The listing builds one solid part. Answer for the finished solid, in the listing's coordinates (mm). Face numbers are marked on the shaded views. A direction names the side the tool comes from. Give positions to 0.01 mm unless a question says otherwise; leave off trailing zeros. Write each loop counter-clockwise with the first axis right and the second up, starting at its lowest first coordinate (ties: lowest second). Pieces come first, ordered by that corner, then holes. Notation, with made-up numbers: (6.5, -20) -> (41.5, -20) arc R13 ccw to (41.5, -11) -> close; hole circle Ø11 at (21, -38.5). An arc over 180 degrees is marked (long way). Use CSV: the item, a comma, the result in double quotes. Start each with the question number.
from build123d import *

# Parameters (mm, degrees)
BASE_EXTRUDE_DEPTH      = 38.1
SKETCH2_R               = 2.3495
MOTOR_HOLE_CUT_DEPTH    = 48.603828628
SKETCH3_R               = 2.3495
MOUNTING_HOLE_CUT_DEPTH = 47.6627796
CORNER_FILLETS_R        = 6.35


with BuildPart() as part:
    # Sketch1 → Base Extrude (new body)
    with BuildSketch(Plane(origin=(0, 0, 0), x_dir=(1, 0, 0), z_dir=(0, 1, 0))):
        Polygon((0, 0), (24.13, 0), (24.13, -3.81), (11.7475, -3.81), (5.08, -6.6548), (5.08, -19.05), (0, -19.05), align=None)
    extrude(amount=BASE_EXTRUDE_DEPTH)

    # Sketch2 → Motor Hole Cut (cut, through all)
    with BuildSketch(Plane.XY.offset(3.81)):
        with Locations((17.697323232, 6.35)):
            Circle(SKETCH2_R)
        with Locations((17.78, 19.05)):
            Circle(SKETCH2_R)
        with Locations((17.78, 31.75)):
            Circle(SKETCH2_R)
    extrude(amount=-MOTOR_HOLE_CUT_DEPTH, mode=Mode.SUBTRACT)

    # Sketch3 → Mounting Hole Cut (cut, through all)
    with BuildSketch(Plane(origin=(5.08, 0, 0), x_dir=(0, 0, -1), z_dir=(1, 0, 0))):
        with Locations((-12.7, 31.75)):
            Circle(SKETCH3_R)
        with Locations((-12.7, 19.05)):
            Circle(SKETCH3_R)
        with Locations((-12.7, 6.35)):
            Circle(SKETCH3_R)
    extrude(amount=-MOUNTING_HOLE_CUT_DEPTH, mode=Mode.SUBTRACT)

    # Corner Fillets
    corner_fillets_edges = [part.edges().sort_by_distance(p)[0] for p in [
        (24.13, 38.1, 1.905),
        (24.13, 0, 1.905),
        (2.54, 38.1, 19.05),
        (2.54, 0, 19.05),
    ]]
    fillet(corner_fillets_edges, radius=CORNER_FILLETS_R)


solid = part.part
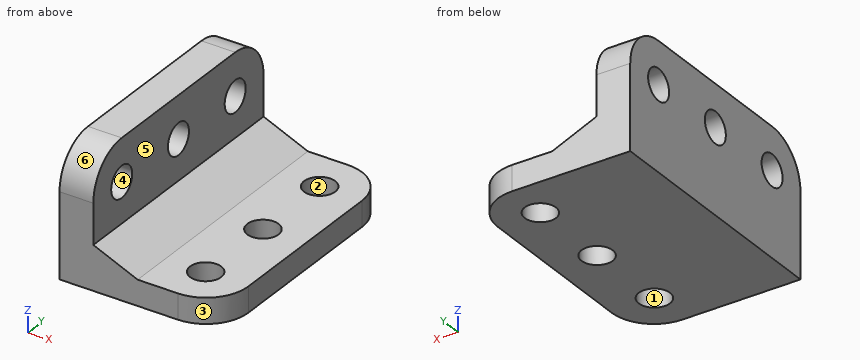
Q1. Section A-A on y = 19.05 is taken. Give the vertices of the cut face in (x, z), then the cut area to 3 significant figures.
Q2. For the marked faces 5 and 6, determine the directions among +Z, -Z, +X, -X, +Y, -Y from which every point of the face is accessible in a straight line to the end or side of a thin tool.
Q3. The mould has two halves that part along X. Classify the marked faces 1, 2, 3 and 4: +X half, -X half, draft (parallel to the pull), parting line (faces both ways), or undercut.
Q4. Section B-B on x = 3 is taken. Give the vertices of the cut face in (y, z), then the cut area to 3 significant figures.
Q5. Flat-ended cylindrical pins translate along their axes: pin 1 Ø3 at (y, z) = (26, 16) entering from +X; pin 2 Ø8 at (y, z) = (30, 8.5) entering from +X; pin 3 Ø5.5 at (x, y) = (17.78, 31.75) entering from +Z; pin 4 Ø4 at (y, z) = (6.35, 12.7) entering from -X. Find the tip coordinate at first contact, or state that the pin passes through.
Q6. Section D-D on y = 13 is taken. Give the vertices of the cut face in (x, z), then the cut area to 3 significant figures.
Q7. Straight lines are drawn through the part: L1, parallel to Y at x = 17.78, z = 2.35; L2, parallel to X at y = 10.5, z = 9.75; L3, parallel to Z at x = 22.25, y = 20.5. For each, find the intervals that lie inside material, in ascending order.
Q8. Section C-C on z = 1.5 is taken. Give the vertices of the cut face in (x, y).
Output:
1,outline,"(0, 0) -> (15.43, 0) -> (15.43, 3.81) -> (11.75, 3.81) -> (5.08, 6.65) -> (5.08, 10.35) -> (0, 10.35) -> close; (0, 15.05) -> (5.08, 15.05) -> (5.08, 19.05) -> (0, 19.05) -> close; (20.13, 0) -> (24.13, 0) -> (24.13, 3.81) -> (20.13, 3.81) -> close"
1,area,"137 mm²"
2,face 5,"+Z, +X, +Y, -Y"
2,face 6,"+Z, +X, -X, -Y"
3,face 1,"undercut"
3,face 2,"undercut"
3,face 3,"+X half"
3,face 4,"draft"
4,outline,"(0, 0) -> (38.1, 0) -> (38.1, 12.7) arc R6.35 ccw to (31.75, 19.05) -> (6.35, 19.05) arc R6.35 ccw to (0, 12.7) -> close; hole circle Ø4.7 at (6.35, 12.7); hole circle Ø4.7 at (19.05, 12.7); hole circle Ø4.7 at (31.75, 12.7)"
4,area,"656 mm²"
5,pin 1,"x = 5.08"
5,pin 2,"x = 10.13"
5,pin 3,"z = 3.81"
5,pin 4,"through"
6,outline,"(0, 0) -> (24.13, 0) -> (24.13, 3.81) -> (11.75, 3.81) -> (5.08, 6.65) -> (5.08, 19.05) -> (0, 19.05) -> close"
6,area,"179 mm²"
7,L1,"0 to 4, 8.7 to 16.7, 21.4 to 29.4, 34.1 to 38.1"
7,L2,"0 to 5.08"
7,L3,"0 to 3.81"
8,outline,"(0, 0) -> (17.78, 0) arc R6.35 ccw to (24.13, 6.35) -> (24.13, 31.75) arc R6.35 ccw to (17.78, 38.1) -> (0, 38.1) -> close; hole circle Ø4.7 at (17.7, 6.35); hole circle Ø4.7 at (17.78, 19.05); hole circle Ø4.7 at (17.78, 31.75)"
